```python
from build123d import *

# Parameters (mm, degrees)
AUFSATZ_LINEAR_AUSTRAGEN1_DEPTH    = 20
SKIZZE2_R                          = 1.6499999999999988
SKIZZE2_R_2                        = 2.65
SKIZZE2_R_3                        = 2.250000000000001
SCHNITT_LINEAR_AUSTRAGEN1_DEPTH    = 3
SKIZZE3_R                          = 2.250000000000001
SKIZZE3_R_2                        = 1.6499999999999988
AUFSATZ_LINEAR_AUSTRAGEN2_DEPTH    = 1
SKIZZE5_W                          = 1.9999999999999998
SKIZZE5_H                          = 2
SCHNITT_LINEAR_AUSTRAGEN2_DEPTH    = 1
K_RPER_VERSCHIEBEN_KOPIEREN1_ANGLE = 90.00000000007478


with BuildPart() as part:
    # Skizze1 → Aufsatz-Linear austragen1 (new body)
    with BuildSketch(Plane.XY):
        Polygon((0, 0), (51.099999999999994, 0), (51.1, 2.5), (45, 2.499999999999999), (45, 3.0000000000000058), (6e-16, 3), align=None)
    extrude(amount=AUFSATZ_LINEAR_AUSTRAGEN1_DEPTH)

    # Skizze2 → Schnitt-Linear austragen1 (cut)
    with BuildSketch(Plane.XZ):
        with Locations(Location((26.699999999999996, 9.999999999999998, 0), (0, 0, 270))):
            Circle(SKIZZE2_R)
        with Locations(Location((40.99999999999999, 10, 0), (0, 0, 270))):
            Circle(SKIZZE2_R_2)
        with Locations(Location((13.699999999999996, 10, 0), (0, 0, 270))):
            Circle(SKIZZE2_R_3)
        with Locations(Location((5.699999999999995, 9.999999999999998, 0), (0, 0, 270))):
            Circle(SKIZZE2_R_3)
    extrude(amount=-SCHNITT_LINEAR_AUSTRAGEN1_DEPTH, mode=Mode.SUBTRACT)

    # Skizze3 → Aufsatz-Linear austragen2 (add)
    with BuildSketch(Plane(origin=(-3.8e-16, 3, 0), x_dir=(1, 1.2e-16, 0), z_dir=(-1.2e-16, 1, 0))):
        Polygon((39.887048957087536, 0), (9.5e-16, 0), (9.5e-16, -8), (-1.9999999999999987, -8), (-1.9999999999999987, -10), (9.5e-16, -10), (9.5e-16, -20), (39.887048957087536, -19.99999999999999), (31.39999999999999, -15.1), (31.39999999999999, -4.900000000000001), align=None)
        with Locations((5.699999999999995, -9.999999999999998)):
            Circle(SKIZZE3_R, mode=Mode.SUBTRACT)
        with Locations((13.699999999999996, -10)):
            Circle(SKIZZE3_R, mode=Mode.SUBTRACT)
        with Locations((26.699999999999996, -9.999999999999998)):
            Circle(SKIZZE3_R_2, mode=Mode.SUBTRACT)
    extrude(amount=AUFSATZ_LINEAR_AUSTRAGEN2_DEPTH)

    # Skizze4 → Schnitt-Rotation3 (revolve, cut)
    with BuildSketch(Plane.XY.offset(10), mode=Mode.PRIVATE) as schnitt_rotation3_sk:
        Polygon((23.699999999999996, 3.9999999999999964), (23.699999999999996, 1.699999999999991), (25.199999999999992, 0.2), (26.699999999999996, 0.2000000000000001), (26.699999999999996, 3.9999999999999964), align=None)
    revolve(schnitt_rotation3_sk.sketch.rotate(Axis((26.699999999999996, 0.2000000000000001, 10), (0, 1, 0)), 270), axis=Axis((26.699999999999996, 0.2000000000000001, 10), (0, 1, 0)), mode=Mode.SUBTRACT)

    # Skizze5 → Schnitt-Linear austragen2 (cut)
    with BuildSketch(Plane(origin=(0, 4, 0), x_dir=(1, 0, 0), z_dir=(0, 1, 0))):
        with Locations((-1, -9)):
            Rectangle(SKIZZE5_W, SKIZZE5_H)
    extrude(amount=-SCHNITT_LINEAR_AUSTRAGEN2_DEPTH, mode=Mode.SUBTRACT)


with BuildPart() as part_1:
    # Körper-Verschieben/Kopieren1: moved
    add(part.part.rotate(Axis((0, 1.500000000000004, 9.999999999999998), (1, 0, 0)), K_RPER_VERSCHIEBEN_KOPIEREN1_ANGLE))


solid = part_1.part
```
Here's how the part is built. I have some questions about the finished solid (model axes, mm). A direction names the side the tool comes from. Coordinates: 2 decimals unless noted, no trailing zeros. Order: outer loops, then holes, each group sorted by start corner. A loop starts at its lowest first (then second) coordinate and runs counter-clockwise, first axis right, second up. Notation, with made-up numbers: (3, 4.5) - (24, 4.5) arc R25 ccw to (24, 36.5) - close; hole circle Ø5 at (-14, -10.75). An arc over 180 degrees is marked (long way). One line per question, with ' | ' between items. Start each with the question number.
1. If we section it at A-A (x = 13.7): Write out the boundary of the cut face in (y, z), and give its area (3 significant figures).
2. If we section it at C-C (x = 26.7): Write out the boundary of the cut face in (y, z), and give its area (3 significant figures).
3. Please list where these lines run through material, in increasing order: line 1 along X through (y, z) = (1.5, 8.65); line 2 along X through (y, z) = (1.5, 9.85); line 3 along Y through (x, z) = (13.7, 11.3). Write a range as [from, to].
4. If we section it at D-D (y = -5.5): Write out the boundary of the cut face in (x, z), and give its area (3 significant figures).
5. If we section it at B-B (y = 1.5): Write out the boundary of the cut face in (x, z).
6. Which directions (+Z, -Z, +X, -X, +Y, -Y) give clear straight access to the entire face, cutting with the end or side of a thin tool? Please do faces 1 (the flat face through (48, 2, 11)), 2 (the cylindrical face through (29.63, 0.85, 11.33)), 3 (the flat face through (31.4, 1, 12)), 4 (the cylindrical face through (43.63, 1.16, 9.98)).
7. I'm going to push flat-ended pins straight in: pin 1 Ø7 at (x, y) = (41, 1.5) entering from -Z; pin 2 Ø5.5 at (x, y) = (26.7, 1.5) entering from +Z; pin 3 Ø2.5 at (x, y) = (13.7, 1.5) entering from +Z; pin 4 Ø1.1 at (y, z) = (-0.5, 12) entering from +X. Where does each tip first touch, or does it pass through?
8. If we mould it in two halves opening along Y, with no side actions, what happens to faces 5 (the flat face through (25, -8.5, 10)), 6 (the flat face through (38, 2, 11.5)), 7 (the flat face through (25, 4, 8.5))? For each: released by +Y, released by -Y, zero draft, split by the parting line, or undercut.
Model answer:
1) outline: (-8.5, 8.5) - (-0.75, 8.5) - (-0.75, 12.5) - (-8.5, 12.5) - close; (3.75, 8.5) - (11.5, 8.5) - (11.5, 12.5) - (3.75, 12.5) - close | area: 62.0 mm²
2) outline: (-8.5, 8.5) - (-0.15, 8.5) - (-0.15, 8.85) - (-1.5, 10.2) - (-1.5, 12.5) - (-8.5, 12.5) - close; (3.15, 8.5) - (11.5, 8.5) - (11.5, 12.5) - (4.5, 12.5) - (4.5, 10.2) - (3.15, 8.85) - close | area: 58.8 mm²
3) line 1: x = [0, 3.45], [7.95, 11.45], [15.95, 25.05], [28.35, 38.35], [43.65, 51.1] | line 2: x = [0, 3.45], [7.95, 11.45], [15.95, 24.05], [29.35, 38.35], [43.65, 51.1] | line 3: y = [-8.5, -0.75], [3.75, 11.5]
4) outline: (0, 8.5) - (51.1, 8.5) - (51.1, 11) - (45, 11) - (45, 11.5) - (34.69, 11.5) - (34.69, 12.5) - (0, 12.5) - close | area: 185 mm²
5) outline: (0, 8.5) - (3.45, 8.5) - (3.45, 12.5) - (0, 12.5) - close; (7.95, 8.5) - (11.45, 8.5) - (11.45, 12.5) - (7.95, 12.5) - close; (15.95, 8.5) - (25.05, 8.5) - (25.05, 8.85) - (23.7, 10.2) - (23.7, 12.5) - (15.95, 12.5) - close; (28.35, 8.5) - (38.35, 8.5) - (38.35, 11.5) - (31.4, 11.5) - (31.4, 12.5) - (29.7, 12.5) - (29.7, 10.2) - (28.35, 8.85) - close; (43.65, 8.5) - (51.1, 8.5) - (51.1, 11) - (45, 11) - (45, 11.5) - (43.65, 11.5) - close
6) face 1: +Z, +X, +Y, -Y | face 2: +Z | face 3: +Z, +X | face 4: +Z, -Z
7) pin 1: stops at z = 8.5 | pin 2: stops at z = 9.95 | pin 3: passes through | pin 4: stops at x = 45
8) face 5: released by -Y | face 6: undercut | face 7: zero draft
